Work out the finished part from the listing and answer in its coordinate system (mm). Give positions to 0.01 mm unless a question says otherwise; leave off trailing zeros. Loops run counter-clockwise (first coordinate to the right, second up) from the corner with the lowest first, then second, coordinate; pieces in that order, holes last. Notation, with made-up numbers: M 15,89 L 69,89 A15 ccw 69,101 Z; hole C 53.25,0 d10. An arc over 180 degrees is marked long. Write item = value, one per line. Start each with the question number.
1. Section C-C on y = 2 is taken. Determine the outline of the cut face in (x, z), plus the area to 3 significant figures.
2. Section D-D on y = 14.5 is taken. Determine the outline of the cut face in (x, z), plus the area to 3 significant figures.
3. Consider L1, parallel to X at y = -1, z = 1.35; L2, parallel to X at y = -7, z = 2.15; L3, parallel to X at y = 13.5, z = 1.15. Determine where each line is inside the solid, lowest interval first. Write a range as [from, to].
4. Flat-ended cylindrical pins translate along their axes: pin 1 Ø1.6 at (x, z) = (-20.5, 0.5) entering from -Y; pin 2 Ø1.8 at (x, y) = (20.5, -0.5) entering from +Z; pin 3 Ø0.8 at (y, z) = (1, 2.5) entering from -X. Find the tip coordinate at first contact, or state that the pin passes through.
5. Section A-A on z = 0.45 is taken. Determine the outline of the cut face in (x, y).
6. Section B-B on y = 9.5 is taken. Determine the outline of the cut face in (x, z).
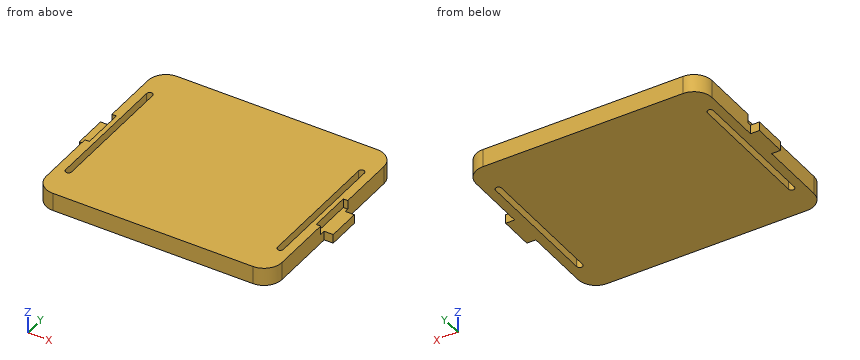
```python
from build123d import *

# Parameters (mm, degrees)
F2_DEPTH = 3
F1_W     = 1.5
F1_H     = 5.6522476953
F3_DEPTH = 1.5


with BuildPart() as f2:
    # F1 (on Top) → F2 (new body)
    with BuildSketch(Plane.XY):
        with BuildLine():
            Line((16.665947184, 16.6212058179), (-16.665947184, 16.6212058179))
            ThreePointArc((-16.665947184, 16.6212058179), (-18.7872675275, 15.7425261615), (-19.665947184, 13.6212058179))
            Line((-19.665947184, 13.6212058179), (-19.665947184, 3.9769788273))
            Line((-19.665947184, 3.9769788273), (-18.915947184, 3.9769788273))
            Line((-18.915947184, 3.9769788273), (-18.915947184, -3.2694519032))
            Line((-18.915947184, -3.2694519032), (-19.665947184, -3.2694519032))
            Line((-19.665947184, -3.2694519032), (-19.665947184, -13.6212058179))
            ThreePointArc((-19.665947184, -13.6212058179), (-18.7872675275, -15.7425261615), (-16.665947184, -16.6212058179))
            Line((-16.665947184, -16.6212058179), (16.665947184, -16.6212058179))
            ThreePointArc((16.665947184, -16.6212058179), (18.7872675275, -15.7425261615), (19.665947184, -13.6212058179))
            Line((19.665947184, -13.6212058179), (19.665947184, -3.2694519032))
            Line((19.665947184, -3.2694519032), (18.915947184, -3.2694519032))
            Line((18.915947184, -3.2694519032), (18.915947184, 3.9769788273))
            Line((18.915947184, 3.9769788273), (19.665947184, 3.9769788273))
            Line((19.665947184, 3.9769788273), (19.665947184, 13.6212058179))
            ThreePointArc((19.665947184, 13.6212058179), (18.7872675275, 15.7425261615), (16.665947184, 16.6212058179))
        make_face()
        with BuildLine():
            Line((-18.165947184, -10.8459210023), (-18.165947184, 10.8459210023))
            ThreePointArc((-18.165947184, 10.8459210023), (-17.665947184, 11.3459210023), (-17.165947184, 10.8459210023))
            Line((-17.165947184, 10.8459210023), (-17.165947184, -10.8459210023))
            ThreePointArc((-17.165947184, -10.8459210023), (-17.665947184, -11.3459210023), (-18.165947184, -10.8459210023))
        make_face(mode=Mode.SUBTRACT)
        with BuildLine():
            ThreePointArc((17.165947184, 10.8459210023), (17.665947184, 11.3459210023), (18.165947184, 10.8459210023))
            Line((18.165947184, 10.8459210023), (18.165947184, -10.8459210023))
            ThreePointArc((18.165947184, -10.8459210023), (17.665947184, -11.3459210023), (17.165947184, -10.8459210023))
            Line((17.165947184, -10.8459210023), (17.165947184, 10.8459210023))
        make_face(mode=Mode.SUBTRACT)
    extrude(amount=F2_DEPTH)

    # F1 (on Top) → F3 (join)
    with BuildSketch(Plane.XY):
        with Locations((-20.415947184, 0.5000088131)):
            Rectangle(F1_W, F1_H)
        Polygon((-18.915947184, 3.9769788273), (-19.665947184, 3.9769788273), (-19.665947184, 3.3261326607), (-19.665947184, -2.3261150345), (-19.665947184, -3.2694519032), (-18.915947184, -3.2694519032), align=None)
        Polygon((19.665947184, 3.3261326607), (19.665947184, 3.9769788273), (18.915947184, 3.9769788273), (18.915947184, -3.2694519032), (19.665947184, -3.2694519032), (19.665947184, -2.3261150345), align=None)
        with Locations((20.415947184, 0.5000088131)):
            Rectangle(F1_W, F1_H)
    extrude(amount=F3_DEPTH)


solid = f2.part
```
Verdict:
q1.outline = M -21.17,0 L -18.17,0 L -18.17,3 L -18.92,3 L -18.92,1.5 L -21.17,1.5 Z; M -17.17,0 L 17.17,0 L 17.17,3 L -17.17,3 Z; M 18.17,0 L 21.17,0 L 21.17,1.5 L 18.92,1.5 L 18.92,3 L 18.17,3 Z
q1.area = 114 mm2
q2.outline = M -19.53,0 L 19.53,0 L 19.53,3 L -19.53,3 Z
q2.area = 117 mm2
q3.L1 = [-21.17, -18.17], [-17.17, 17.17], [18.17, 21.17]
q3.L2 = [-19.67, -18.17], [-17.17, 17.17], [18.17, 19.67]
q3.L3 = [-19.67, 19.67]
q4.pin_1 = -2.33
q4.pin_2 = 1.5
q4.pin_3 = -18.92
q5.outline = M -21.17,-2.33 L -19.67,-2.33 L -19.67,-13.62 A3 ccw -16.67,-16.62 L 16.67,-16.62 A3 ccw 19.67,-13.62 L 19.67,-2.33 L 21.17,-2.33 L 21.17,3.33 L 19.67,3.33 L 19.67,13.62 A3 ccw 16.67,16.62 L -16.67,16.62 A3 ccw -19.67,13.62 L -19.67,3.33 L -21.17,3.33 Z; hole M -18.17,-10.85 A0.5 ccw -17.17,-10.85 L -17.17,10.85 A0.5 ccw -18.17,10.85 Z; hole M 17.17,-10.85 A0.5 ccw 18.17,-10.85 L 18.17,10.85 A0.5 ccw 17.17,10.85 Z
q6.outline = M -19.67,0 L -18.17,0 L -18.17,3 L -19.67,3 Z; M -17.17,0 L 17.17,0 L 17.17,3 L -17.17,3 Z; M 18.17,0 L 19.67,0 L 19.67,3 L 18.17,3 Z
